from build123d import *

# Parameters (mm, degrees)
SKETCH1_W                = 70
SKETCH1_H                = 20
BOSS_EXTRUDE1_DEPTH      = 5
SKETCH2_W                = 90
SKETCH2_H                = 20
BOSS_EXTRUDE2_DEPTH      = 3
BOSS_EXTRUDE3_DEPTH      = 28
CUT_EXTRUDE1_DEPTH       = 59.489315264
FILLET1_R                = 2
FILLET2_R                = 2
M3_CLEARANCE_HOLE1_D     = 3.4
M3_CLEARANCE_HOLE1_DEPTH = 10
M3_CLEARANCE_HOLE1_TIP   = 1.021463052


with BuildPart() as part:
    # Sketch1 → Boss-Extrude1 (new body)
    with BuildSketch(Plane(origin=(0, 0, 0), x_dir=(1, 0, 0), z_dir=(0, 1, 0))):
        Rectangle(SKETCH1_W, SKETCH1_H)
    extrude(amount=BOSS_EXTRUDE1_DEPTH)

    # Sketch2 → Boss-Extrude2 (add)
    with BuildSketch(Plane.XZ):
        Rectangle(SKETCH2_W, SKETCH2_H)
    extrude(amount=BOSS_EXTRUDE2_DEPTH)

    # Sketch4 → Boss-Extrude3 (add)
    with BuildSketch(Plane(origin=(0, 5, 0), x_dir=(1, 0, 0), z_dir=(0, 1, 0))):
        with BuildLine():
            Line((17.5, 10), (-17.5, 10))
            ThreePointArc((-17.5, 10), (0, -7.5), (17.5, 10))
        make_face()
    extrude(amount=BOSS_EXTRUDE3_DEPTH)

    # Sketch6 → Cut-Extrude1 (cut, through all)
    with BuildSketch(Plane(origin=(0, 33, 0), x_dir=(1, 0, 0), z_dir=(0, 1, 0))):
        with BuildLine():
            Line((15.370426149, 8), (-15.370426149, 8))
            ThreePointArc((-15.370426149, 8), (0, -5.5), (15.370426149, 8))
        make_face()
    extrude(amount=-CUT_EXTRUDE1_DEPTH, mode=Mode.SUBTRACT)

    # Fillet1
    fillet1_edges = [part.edges().sort_by_distance(p)[0] for p in [
        (0, 33, 5.5),
        (0, 33, -8),
    ]]
    fillet(fillet1_edges, radius=FILLET1_R - 0.0001)  # a hair under: the kernel refuses the full size

    # Fillet2
    fillet2_edges = [part.edges().sort_by_distance(p)[0] for p in [
        (0, -3, 5.5),
        (0, -3, -8),
    ]]
    fillet(fillet2_edges, radius=FILLET2_R - 0.0001)  # a hair under: the kernel refuses the full size

    # M3 Clearance Hole1
    with Locations(Plane(origin=(0, 0, 0), x_dir=(1, 0, 0), z_dir=(0, 1, 0))):
        with Locations((-40, 6), (-40, -6), (40, 6), (40, -6)):
            Hole(M3_CLEARANCE_HOLE1_D / 2, depth=M3_CLEARANCE_HOLE1_DEPTH)
            with Locations((0, 0, -(M3_CLEARANCE_HOLE1_DEPTH + M3_CLEARANCE_HOLE1_TIP / 2))):  # 118° drill point
                Cone(0, M3_CLEARANCE_HOLE1_D / 2, M3_CLEARANCE_HOLE1_TIP, mode=Mode.SUBTRACT)


solid = part.part
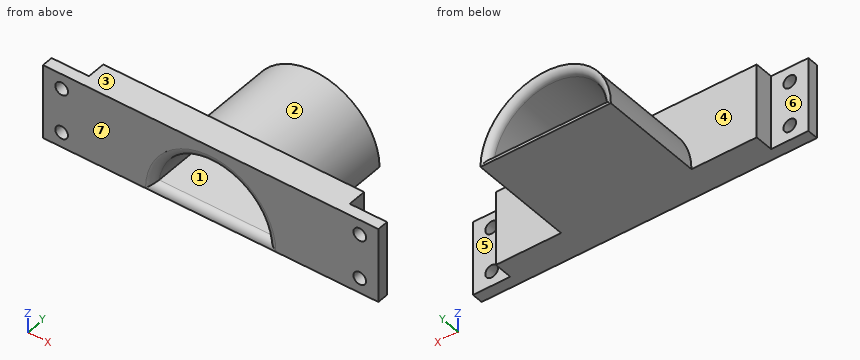
Part model, mm, in its own coordinate system. Face numbers are marked on the shaded views. A direction names the side the tool comes from. Give positions to 0.01 mm unless a question says otherwise; leave off trailing zeros. Write each loop counter-clockwise with the first axis right and the second up, starting at its lowest first coordinate (ties: lowest second). Pieces come first, ordered by that corner, then holes.
1) Pin check, flat tips, straight feed: pin 1 (10 mm diameter, centred on x = 36, z = 6.5, fed in from +Y); pin 2 (4.5 mm diameter, centred on x = -40, z = -6, fed in from +Y); pin 3 (5 mm diameter, centred on x = -5, y = 13, fed in from +Z); pin 4 (2 mm diameter, centred on x = 40, z = 6, fed in from -Y). Stop position of each tip, or through.
Resolved:
pin 1: stops at y = 5
pin 2: stops at y = 0
pin 3: stops at z = 7.32
pin 4: passes through
2) Two-plate mould, pull along X, no slides. Class the marked faces 1, 2 and 3: released by +X, released by -X, zero draft, split by the parting line, or undercut.
Resolved:
face 1: undercut
face 2: split by the parting line
face 3: zero draft
3) Probe L1, parallel to X at y = -1.8, z = 6; L2, parallel to Z at x = 40, y = -0.7; L3, parallel to X at y = -2.4, z = -6. List the from-to ranges inside material, lowest first.
Resolved:
L1: x = -45 to -41.7, -38.3 to 38.3, 41.7 to 45
L2: z = -10 to -7.7, -4.3 to 4.3, 7.7 to 10
L3: x = -45 to -41.7, -38.3 to -15.57, 15.57 to 38.3, 41.7 to 45
4) Which spindle directions (+Z, -Z, +X, -X, +Y, -Y) get a long thin tool onto all of the face, cutting with end or side? Do the marked faces 4, 5, 6 and 7. Say none if no direction does.
Resolved:
face 4: +Z, +Y
face 5: +Z, -Z, +X, +Y
face 6: +Z, -Z, -X, +Y
face 7: +Z, -Z, +X, -X, -Y
5) Cut at C-C on x = -40. Write the cut outline in (y, z).
Resolved:
outline: (-3, -10) - (0, -10) - (0, -7.7) - (-3, -7.7) - close; (-3, -4.3) - (0, -4.3) - (0, 4.3) - (-3, 4.3) - close; (-3, 7.7) - (0, 7.7) - (0, 10) - (-3, 10) - close
6) Cut at B-B on y = 3. Write the cut outline in (x, z), then the cut area to 3 significant figures.
Resolved:
outline: (-35, -10) - (35, -10) - (35, 10) - (-35, 10) - close; hole (-15.37, -8) - (15.37, -8) arc R15.5 ccw to start
area: 1,080 mm2
7) Cut at D-D on z = -6. State how many separate pieces and enclosed holes the cut face has, then the cut area to 3 significant figures.
Resolved:
separate pieces: 4
enclosed holes: 0
area: 472 mm2
